```python
from build123d import *

# Parameters (mm, degrees)
SKETCH1_R           = 60
BOSS_EXTRUDE1_DEPTH = 1
FILLET1_R           = 2


with BuildPart() as part:
    # Sketch1 → Boss-Extrude1 (new body)
    with BuildSketch(Plane(origin=(0, 0, 0), x_dir=(1, 0, 0), z_dir=(0, 1, 0))):
        with Locations(Location((0, 0, 0), (0, 0, 270))):
            Circle(SKETCH1_R)
        with BuildLine():
            Line((-29.221443851, 34.221443851), (0, 5))
            Line((0, 5), (29.221443851, 34.221443851))
            ThreePointArc((29.221443851, 34.221443851), (0, -45), (-29.221443851, 34.221443851))
        make_face(mode=Mode.SUBTRACT)
    extrude(amount=BOSS_EXTRUDE1_DEPTH)

    # Fillet1
    fillet1_edges = [part.edges().sort_by_distance(p)[0] for p in [
        (-29.221443851, 0.5, -34.221443851),
        (29.221443851, 0.5, -34.221443851),
        (0, 0.5, -5),
    ]]
    fillet(fillet1_edges, radius=FILLET1_R)


solid = part.part
```
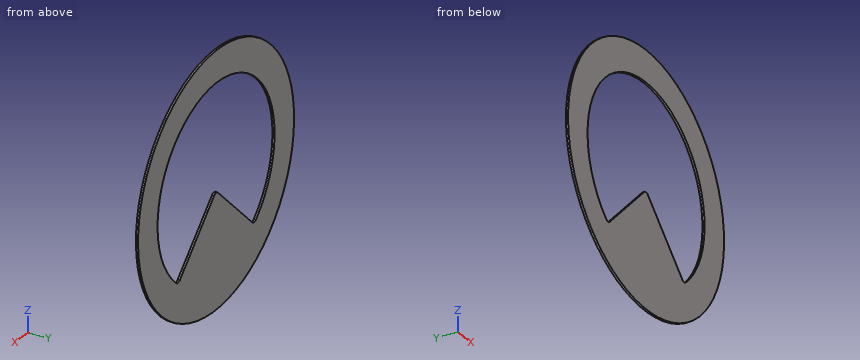
Build history of the part. All positions in model axes, mm. Round coordinates to 2 decimals unless told otherwise and drop trailing zeros. Order: outer loops, then holes, each group sorted by start corner. A loop starts at its lowest first (then second) coordinate and runs counter-clockwise, first axis right, second up. Notation, with made-up numbers: (-28.75, 75) -> (-17.75, 75) arc R29 cw to (-17.75, 112) -> close; hole circle Ø2 at (59.5, 78.5). An arc over 180 degrees is marked (long way). Answer in a Markdown table with one row per item.
1) Band-saw the part on C-C on z = 0. Give the cut face in (x, y), and give its area (3 significant figures).
Values:
| item | result |
|---|---|
| outline | (-60, 0) -> (-45, 0) -> (-45, 1) -> (-60, 1) -> close; (45, 0) -> (60, 0) -> (60, 1) -> (45, 1) -> close |
| area | 30.0 mm2 |
2) Band-saw the part on D-D on z = -14. Give the cut face in (x, y).
Values:
| item | result |
|---|---|
| outline | (-58.34, 0) -> (-42.77, 0) -> (-42.77, 1) -> (-58.34, 1) -> close; (-9, 0) -> (9, 0) -> (9, 1) -> (-9, 1) -> close; (42.77, 0) -> (58.34, 0) -> (58.34, 1) -> (42.77, 1) -> close |
3) Band-saw the part on B-B on y = 0.45. Give the cut face in (x, z), and give its area (3 significant figures).
Values:
| item | result |
|---|---|
| outline | circle Ø120 at (0, 0); hole (-30.66, -32.94) arc R2 ccw to (-27.89, -32.89) -> (-1.41, -6.41) arc R2 cw to (1.41, -6.41) -> (27.89, -32.89) arc R2 ccw to (30.66, -32.94) arc R45 ccw (long way) to start |
| area | 6,230 mm2 |
4) Wall check: L1, parallel to X at y = 0.8, z = 0; L2, parallel to Z at x = -13.5, y = 0.3; L3, parallel to Z at x = -35, y = 0.75. Give the ranges that are in metal, low to high.
Values:
| item | result |
|---|---|
| L1 | -60 to -45, 45 to 60 |
| L2 | -58.46 to -18.5, 42.93 to 58.46 |
| L3 | -48.73 to -28.28, 28.28 to 48.73 |
5) Band-saw the part on A-A on x = 0. Give the cut face in (y, z), and give its area (3 significant figures).
Values:
| item | result |
|---|---|
| outline | (0, -60) -> (1, -60) -> (1, -5.83) -> (0, -5.83) -> close; (0, 45) -> (1, 45) -> (1, 60) -> (0, 60) -> close |
| area | 69.2 mm2 |
